from build123d import *

# Parameters (mm, degrees)
SKETCH1_R           = 7
SKETCH1_R_2         = 2.5
BOSS_EXTRUDE1_DEPTH = 30
SKETCH2_W           = 30
SKETCH2_H           = 58.25
CUT_EXTRUDE1_DEPTH  = 151.539861831
SKETCH3_R           = 7.5
CUT_EXTRUDE2_DEPTH  = 1
CUT_EXTRUDE3_START  = -1
SKETCH4_R           = 7.5
CUT_EXTRUDE3_DEPTH  = 1
SKETCH6_W           = 17.3
SKETCH6_H           = 75
CUT_EXTRUDE4_DEPTH  = 151.539861831
SKETCH7_W           = 46.5
SKETCH7_H           = 1.95
CUT_EXTRUDE5_DEPTH  = 97.065732704
FILLET1_R           = 10


with BuildPart() as part:
    # Sketch1 → Boss-Extrude1 (new, symmetric)
    with BuildSketch(Plane.XY):
        with BuildLine():
            Line((-23.25, 0), (-23.25, 140))
            Line((-23.25, 140), (23.25, 140))
            Line((23.25, 140), (23.25, 0))
            ThreePointArc((23.25, 0), (0, -23.25), (-23.25, 0))
        make_face()
        Circle(SKETCH1_R, mode=Mode.SUBTRACT)
        with Locations((-11.25, 125)):
            Circle(SKETCH1_R_2, mode=Mode.SUBTRACT)
        with Locations((11.25, 125)):
            Circle(SKETCH1_R_2, mode=Mode.SUBTRACT)
        with Locations((11.25, 90)):
            Circle(SKETCH1_R_2, mode=Mode.SUBTRACT)
        with Locations((-11.25, 90)):
            Circle(SKETCH1_R_2, mode=Mode.SUBTRACT)
    extrude(amount=BOSS_EXTRUDE1_DEPTH, both=True)

    # Sketch2 → Cut-Extrude1 (cut, through all)
    with BuildSketch(Plane(origin=(23.25, 0, 0), x_dir=(0, 0, -1), z_dir=(1, 0, 0))):
        with Locations((0, 5.875)):
            Rectangle(SKETCH2_W, SKETCH2_H)
    extrude(amount=-CUT_EXTRUDE1_DEPTH, mode=Mode.SUBTRACT)

    # Sketch3 → Cut-Extrude2 (cut)
    with BuildSketch(Plane.XY.offset(30)):
        Circle(SKETCH3_R)
    extrude(amount=-CUT_EXTRUDE2_DEPTH, mode=Mode.SUBTRACT)

    # Sketch4 → Cut-Extrude3 (cut)
    with BuildSketch(Plane(origin=(0, 0, -30), x_dir=(-1, 0, 0), z_dir=(0, 0, -1)).offset(CUT_EXTRUDE3_START)):
        with Locations(Location((0, 0, 0), (0, 0, 180))):
            Circle(SKETCH4_R)
    extrude(amount=CUT_EXTRUDE3_DEPTH, mode=Mode.SUBTRACT)

    # Sketch6 → Cut-Extrude4 (cut, through all)
    with BuildSketch(Plane(origin=(23.25, 0, 0), x_dir=(0, 0, -1), z_dir=(1, 0, 0))):
        with Locations((-21.35, 102.5)):
            Rectangle(SKETCH6_W, SKETCH6_H)
        with Locations((21.35, 102.5)):
            Rectangle(SKETCH6_W, SKETCH6_H)
    extrude(amount=-CUT_EXTRUDE4_DEPTH, mode=Mode.SUBTRACT)

    # Sketch7 → Cut-Extrude5 (cut, through all)
    with BuildSketch(Plane(origin=(0, 65, 0), x_dir=(1, 0, 0), z_dir=(0, 1, 0))):
        with Locations((0, 11.725)):
            Rectangle(SKETCH7_W, SKETCH7_H)
        with Locations((0, -11.725)):
            Rectangle(SKETCH7_W, SKETCH7_H)
    extrude(amount=CUT_EXTRUDE5_DEPTH, mode=Mode.SUBTRACT)

    # Fillet1
    fillet1_edges = [part.edges().sort_by_distance(p)[0] for p in [
        (23.25, 35, 0),
        (-23.25, 35, 0),
    ]]
    fillet(fillet1_edges, radius=FILLET1_R)


solid = part.part
CAD build for the part. Positions are in the model's coordinates, mm. A direction names the side the tool comes from. Coordinates: 2 decimals unless noted, no trailing zeros. Loops run counter-clockwise (first coordinate to the right, second up) from the corner with the lowest first, then second, coordinate; pieces in that order, holes last. Notation, with made-up numbers: (12.25, 74.25) - (17.25, 74.25) arc R30 ccw to (17.25, 96.25) - close; hole circle Ø3 at (58.5, 40). An arc over 180 degrees is marked (long way). Write item = value, one per line. Start each with the question number.
Q1. Drill centre lines: L1, parallel to X at y = 90, z = 1.5; L2, parallel to Y at x = 11.25, z = 0.5; L3, parallel to Y at x = 0, z = 29.6. Where is each one in solid material? Low to high.
Q2. Flat gauge pins, fed straight in: pin 1 Ø7.5 at (x, y) = (-0.5, -2) entering from -Z; pin 2 Ø15.5 at (x, z) = (-11.5, -24.5) entering from +Y; pin 3 Ø6 at (x, y) = (11.25, 125) entering from +Z; pin 4 Ø21 at (x, z) = (-3.5, 7.5) entering from -Y. Where does each tip first touch, or does it go through?
Q3. Cut at B-B, the plane x = 0. List the corners of the cut face in (y, z), then the cut area to 3 significant figures.
Q4. Cut at D-D, the plane y = -12. List the corners of the cut face in (x, z).
Q5. Pull direction Z, two halves, no side cores. Call faces 1 (the flat face through (0, 102, 10.75)), 2 (the flat face through (0, 102, -10.75)), 3 (the flat face through (0, 10, 15)), 4 (the flat face through (23.25, 71, 0)): pulls with the +Z half, pulls with the -Z half, needs draft (parallel to the pull), parting line crosses it, or undercut.
Q6. Cut at A-A, the plane y = 90. List the corners of the cut face in (x, z).
Q7. Which spindle directions (+Z, -Z, +X, -X, +Y, -Y) get a long thin tool onto all of the face, cutting with end or side? Do faces 5 (the flat face through (-2, 7, -29)), 6 (the flat face through (0, 35, 0)), 7 (the flat face through (0, 140, 0)), 8 (the cylindrical face through (-20.4, 38.01, -0.21)), 9 (the flat face through (7, 2, 29)). Say none if no direction does.
Q8. Cut at C-C, the plane z = 8. List the corners of the cut face in (x, y).
Computed:
q1.L1 = -23.25 to -13.75, -8.75 to 8.75, 13.75 to 23.25
q1.L2 = 35 to 87.5, 92.5 to 122.5, 127.5 to 140
q1.L3 = -23.25 to -7.5, 7.5 to 65
q2.pin_1 = through
q2.pin_2 = 65
q2.pin_3 = 10.75
q2.pin_4 = -23.25
q3.outline = (-23.25, -30) - (-7.5, -30) - (-7.5, -29) - (-7, -29) - (-7, -15) - (-23.25, -15) - close; (-23.25, 15) - (-7, 15) - (-7, 29) - (-7.5, 29) - (-7.5, 30) - (-23.25, 30) - close; (7, -29) - (7.5, -29) - (7.5, -30) - (65, -30) - (65, -10.75) - (140, -10.75) - (140, 10.75) - (65, 10.75) - (65, 30) - (7.5, 30) - (7.5, 29) - (7, 29) - (7, 15) - (35, 15) - (35, -15) - (7, -15) - close
q3.area = 4,740 mm²
q4.outline = (-19.91, -30) - (19.91, -30) - (19.91, -15) - (-19.91, -15) - close; (-19.91, 15) - (19.91, 15) - (19.91, 30) - (-19.91, 30) - close
q5.face_1 = pulls with the +Z half
q5.face_2 = pulls with the -Z half
q5.face_3 = undercut
q5.face_4 = needs draft
q6.outline = (-23.25, -10.75) - (-13.75, -10.75) - (-13.75, 10.75) - (-23.25, 10.75) - close; (-8.75, -10.75) - (8.75, -10.75) - (8.75, 10.75) - (-8.75, 10.75) - close; (13.75, -10.75) - (23.25, -10.75) - (23.25, 10.75) - (13.75, 10.75) - close
q7.face_5 = -Z
q7.face_6 = +X, -X, -Y
q7.face_7 = +Z, -Z, +X, -X, +Y
q7.face_8 = -X, -Y
q7.face_9 = +Z
q8.outline = (-23.25, 45) arc R10 ccw to (-13.25, 35) - (13.25, 35) arc R10 ccw to (23.25, 45) - (23.25, 140) - (-23.25, 140) - close; hole circle Ø5 at (-11.25, 90); hole circle Ø5 at (-11.25, 125); hole circle Ø5 at (11.25, 90); hole circle Ø5 at (11.25, 125)
